from build123d import *

# Parameters (mm, degrees)
SKETCH2_W           = 355.6
SKETCH2_H           = 165.1
SKETCH2_R           = 31.75
SKETCH2_R_2         = 6.35
BOSS_EXTRUDE1_DEPTH = 4.7625
CUT_EXTRUDE1_DEPTH  = 5.7625
CUT_EXTRUDE3_DEPTH  = 5.7625


with BuildPart() as part:
    # Sketch2 → Boss-Extrude1 (new body)
    with BuildSketch(Plane.XY):
        with Locations((95.25, 0)):
            Rectangle(SKETCH2_W, SKETCH2_H)
        Circle(SKETCH2_R, mode=Mode.SUBTRACT)
        with Locations((-54.018973032, 17.551828308)):
            Circle(SKETCH2_R_2, mode=Mode.SUBTRACT)
        with Locations((0, 56.798909535)):
            Circle(SKETCH2_R_2, mode=Mode.SUBTRACT)
        with Locations((54.018973032, 17.551828308)):
            Circle(SKETCH2_R_2, mode=Mode.SUBTRACT)
        with Locations((33.385561371, -45.951283076)):
            Circle(SKETCH2_R_2, mode=Mode.SUBTRACT)
        with Locations((-33.385561371, -45.951283076)):
            Circle(SKETCH2_R_2, mode=Mode.SUBTRACT)
    extrude(amount=BOSS_EXTRUDE1_DEPTH)

    # Sketch3 → Cut-Extrude1 (cut, through all)
    with BuildSketch(Plane.XY.offset(4.7625)):
        with BuildLine():
            Line((149.225, -9.525), (130.175, -9.525))
            ThreePointArc((130.175, -9.525), (127, -6.35), (130.175, -3.175))
            Line((130.175, -3.175), (149.225, -3.175))
            ThreePointArc((149.225, -3.175), (152.4, -6.35), (149.225, -9.525))
        make_face()
        with BuildLine():
            Line((250.825, -9.525), (231.775, -9.525))
            ThreePointArc((231.775, -9.525), (228.6, -6.35), (231.775, -3.175))
            Line((231.775, -3.175), (250.825, -3.175))
            ThreePointArc((250.825, -3.175), (254, -6.35), (250.825, -9.525))
        make_face()
        with BuildLine():
            Line((238.125, -60.325), (219.075, -60.325))
            ThreePointArc((219.075, -60.325), (215.9, -57.15), (219.075, -53.975))
            Line((219.075, -53.975), (238.125, -53.975))
            ThreePointArc((238.125, -53.975), (241.3, -57.15), (238.125, -60.325))
        make_face()
        with BuildLine():
            Line((142.875, -53.975), (161.925, -53.975))
            ThreePointArc((161.925, -53.975), (165.1, -57.15), (161.925, -60.325))
            Line((161.925, -60.325), (142.875, -60.325))
            ThreePointArc((142.875, -60.325), (139.7, -57.15), (142.875, -53.975))
        make_face()
    extrude(amount=-CUT_EXTRUDE1_DEPTH, mode=Mode.SUBTRACT)

    # Sketch4 → Cut-Extrude3 (cut, through all)
    with BuildSketch(Plane.XY.offset(4.7625)):
        with BuildLine():
            Line((247.65, 28.575), (247.65, 50.8))
            ThreePointArc((247.65, 50.8), (245.790128061, 55.290128061), (241.3, 57.15))
            Line((241.3, 57.15), (112.395, 57.15))
            ThreePointArc((112.395, 57.15), (107.904871939, 55.290128061), (106.045, 50.8))
            Line((106.045, 50.8), (106.045, 28.575))
            ThreePointArc((106.045, 28.575), (107.904871939, 24.084871939), (112.395, 22.225))
            Line((112.395, 22.225), (241.3, 22.225))
            ThreePointArc((241.3, 22.225), (245.790128061, 24.084871939), (247.65, 28.575))
        make_face()
    extrude(amount=-CUT_EXTRUDE3_DEPTH, mode=Mode.SUBTRACT)


solid = part.part
Here's how the part is built. I have some questions about the finished solid (model axes, mm). A direction names the side the tool comes from. Round coordinates to 2 decimals unless told otherwise and drop trailing zeros. Order: outer loops, then holes, each group sorted by start corner. A loop starts at its lowest first (then second) coordinate and runs counter-clockwise, first axis right, second up. Notation, with made-up numbers: M 64.25,47.5 L 118.25,47.5 A22 ccw 118.25,85.5 Z; hole C -17.75,71.5 d9. An arc over 180 degrees is marked long. Return JSON: item names as keys, results as strings. Group by question number.
1. Please list where these lines run through material, in increasing order: probe 1 along Y at (x, z) = (221, 0.75) (3 decimals); probe 2 along X at (y, z) = (38, 4.15) (3 decimals); probe 3 along Y at (x, z) = (171, 2.3) (3 decimals).
2. If we mould it in two halves opening along Y, with no side actions, what happens to faces 3 (the face through (-48.153, 15.12, 2.348)), 4 (the face through (93, 1, 0))? For each: pulls with the +Y half, pulls with the -Y half, needs draft (parallel to the pull), parting line crosses it, or undercut.
3. If we section it at C-C on x = 0: List the corners of the cut face in (y, z) for me.
4. If we section it at D-D on y = 0: List the corners of the cut face in (x, z) for me, then the cut area to 3 significant figures.
5. On a 3-axis mill with a long thin cutter (end or side, diameter ignored), from which of +Z, -Z, +X, -X, +Y, -Y can I reach the whole of each face in a straight line? I mean faces 1 (the face through (245.74, 24.036, 2.415)), 2 (the face through (93, 1, 4.762)). Say none if no direction works.
6. If we section it at A-A on y = -57.15: List the corners of the cut face in (x, z) for me, then the cut area to 3 significant figures.
Reply:
{
 "1": {"probe 1": "-82.55 to -60.325, -53.975 to 22.225, 57.15 to 82.55", "probe 2": "-82.55 to 106.045, 247.65 to 273.05", "probe 3": "-82.55 to 22.225, 57.15 to 82.55"},
 "2": {"face 3": "undercut", "face 4": "needs draft"},
 "3": {"outline": "M -82.55,0 L -31.75,0 L -31.75,4.76 L -82.55,4.76 Z; M 31.75,0 L 50.45,0 L 50.45,4.76 L 31.75,4.76 Z; M 63.15,0 L 82.55,0 L 82.55,4.76 L 63.15,4.76 Z"},
 "4": {"outline": "M -82.55,0 L -31.75,0 L -31.75,4.76 L -82.55,4.76 Z; M 31.75,0 L 273.05,0 L 273.05,4.76 L 31.75,4.76 Z", "area": "1,390 mm^2"},
 "5": {"face 1": "+Z, -Z", "face 2": "+Z, +X, -X, +Y, -Y"},
 "6": {"outline": "M -82.55,0 L 139.7,0 L 139.7,4.76 L -82.55,4.76 Z; M 165.1,0 L 215.9,0 L 215.9,4.76 L 165.1,4.76 Z; M 241.3,0 L 273.05,0 L 273.05,4.76 L 241.3,4.76 Z", "area": "1,450 mm^2"}
}
